The model under review builds one solid part; all positions refer to its coordinate system, in mm. Face numbers are marked on the shaded views. Give positions to 0.01 mm unless a question says otherwise; leave off trailing zeros. Order: outer loops, then holes, each group sorted by start corner. A loop starts at its lowest first (then second) coordinate and runs counter-clockwise, first axis right, second up. Notation, with made-up numbers: (-32.5, -14) -> (23.5, -14) arc R19 ccw to (23.5, 15) -> close; hole circle Ø5 at (9, -31). An arc over 180 degrees is marked (long way). Answer as a JSON object with one key per item and string values. Group by question number.
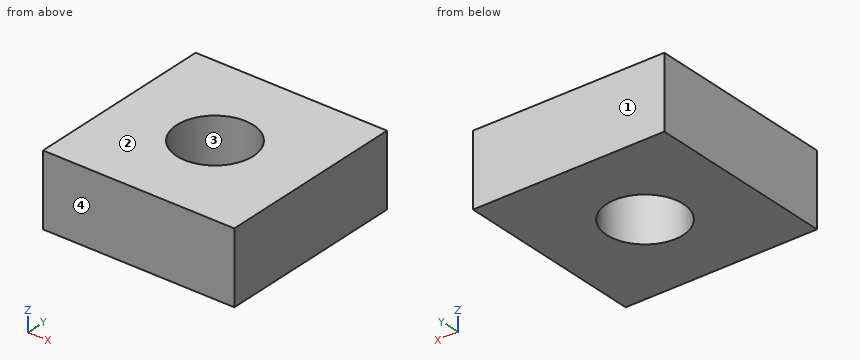
Autodesk Inventor part; units mm, degrees
ref_plane "Plano de trabajo1" through (-9.1, 23, 5.1) normal (0, 0, 1) x (1, 0, 0)
ref_plane "YZ Plane" through (0, 0, 0) normal (1, 0, 0) x (0, 1, 0)
ref_plane "XZ Plane" through (0, 0, 0) normal (0, 1, 0) x (-1, 0, 0)
sketch "Boceto1" plane through (0, 0, 0) normal (0, 0, 1) x (1, 0, 0)
  circle A0 centre (0, 37) radius 2.1
  circle A1 centre (0, -37) radius 2.1
  line L0 (4, 41) -> (4, -41)
  line L1 (-4, 41) -> (4, 41)
  line L2 (-4, -41) -> (-4, 41)
  line L3 (4, -41) -> (-4, -41)
  line L4 (4, 41) -> (-4, 41)
  line L5 (-4, 41) -> (-4, 33)
  line L6 (-4, 33) -> (4, 33)
  line L7 (4, 33) -> (4, 41)
  circle A2 centre (0, 37) radius 1.6
  line L8 (0, 0) -> (0, 33)
  line L9 (4, 33) -> (-4, 33)
  line L10 (-4, 33) -> (-4, 23)
  line L11 (-4, 23) -> (4, 23)
  line L12 (4, 23) -> (4, 33)
  dimension "d2" = 3.2
ref_plane "Plano de trabajo1" through (-9.1, 23, 5.1) normal (0, 0, 1) x (1, 0, 0)
extrude "Extrusión1" add sketch "Boceto1" along normal blind 3 contours A0 | L0 L6 L2 L1
properties part number "Soporte gomas"
1. Take a section at A-A on y = 37. Give the boundary of the cut face in (x, z).
2. For probe 1 along Y at (x, z) = (0, 1.8); probe 2 along X at (y, z) = (36.75, 1.4); probe 3 along X at (y, z) = (36.25, 0.95), list the stretches that pass through material, from the lowest coordinate up. Write a range as [from, to].
3. Take a section at C-C on z = 1.8. Give the boundary of the cut face in (x, y).
4. Take a section at B-B on x = 0. Give the boundary of the cut face in (y, z).
5. Draft analysis for pull direction Y (two halves, no side actions). For the marked faces 1, 2, 3 and 4, state which applies: pulls with the +Y half, pulls with the -Y half, needs draft (parallel to the pull), parting line crosses it, or undercut.
Checks:
{
 "1": {"outline": "(-4, 0) -> (-1.6, 0) -> (-1.6, 3) -> (-4, 3) -> close; (1.6, 0) -> (4, 0) -> (4, 3) -> (1.6, 3) -> close"},
 "2": {"probe 1": "y = [33, 35.4], [38.6, 41]", "probe 2": "x = [-4, -1.58], [1.58, 4]", "probe 3": "x = [-4, -1.41], [1.41, 4]"},
 "3": {"outline": "(-4, 33) -> (4, 33) -> (4, 41) -> (-4, 41) -> close; hole circle Ø3.2 at (0, 37)"},
 "4": {"outline": "(33, 0) -> (35.4, 0) -> (35.4, 3) -> (33, 3) -> close; (38.6, 0) -> (41, 0) -> (41, 3) -> (38.6, 3) -> close"},
 "5": {"face 1": "pulls with the +Y half", "face 2": "needs draft", "face 3": "undercut", "face 4": "pulls with the -Y half"}
}
